from build123d import *

# Parameters (mm, degrees)
SKETCH_1_R          = 10.5
EXTRUDE_1_DEPTH     = 2.5
SKETCH_2_R          = 4.5
EXTRUDE_2_DEPTH     = 3
SKETCH_3_R          = 3
CUT_EXTRUDE_1_DEPTH = 3.5
SKETCH_4_R          = 0.75
CUT_EXTRUDE_2_DEPTH = 4


with BuildPart() as part:
    # 草图1 → 凸台-拉伸1 (new body)
    with BuildSketch(Plane(origin=(0, 0, 0), x_dir=(1, 0, 0), z_dir=(0, 1, 0))):
        with Locations(Location((0, 0, 0), (0, 0, 270))):
            Circle(SKETCH_1_R)
    extrude(amount=EXTRUDE_1_DEPTH)

    # 草图2 → 凸台-拉伸2 (add)
    with BuildSketch(Plane(origin=(0, 2.5, 0), x_dir=(1, 0, 0), z_dir=(0, 1, 0))):
        with Locations(Location((0, 0, 0), (0, 0, 270))):
            Circle(SKETCH_2_R)
    extrude(amount=EXTRUDE_2_DEPTH)

    # 草图3 → 切除-拉伸1 (cut)
    with BuildSketch(Plane(origin=(0, 5.5, 0), x_dir=(1, 0, 0), z_dir=(0, 1, 0))):
        with Locations(Location((0, 0, 0), (0, 0, 270))):
            Circle(SKETCH_3_R)
    extrude(amount=-CUT_EXTRUDE_1_DEPTH, mode=Mode.SUBTRACT)

    # 草图4 → 切除-拉伸2 (cut)
    with BuildSketch(Plane.XZ):
        with Locations(Location((0, 8, 0), (0, 0, 270))):
            Circle(SKETCH_4_R)
        with Locations(Location((3.253893145, 7.308363661, 0), (0, 0, 270))):
            Circle(SKETCH_4_R)
        with Locations(Location((5.945158604, 5.353044851, 0), (0, 0, 270))):
            Circle(SKETCH_4_R)
        with Locations(Location((7.60845213, 2.472135955, 0), (0, 0, 270))):
            Circle(SKETCH_4_R)
        with Locations(Location((7.956175163, -0.836227706, 0), (0, 0, 270))):
            Circle(SKETCH_4_R)
        with Locations(Location((6.92820323, -4, 0), (0, 0, 270))):
            Circle(SKETCH_4_R)
        with Locations(Location((4.702282018, -6.472135955, 0), (0, 0, 270))):
            Circle(SKETCH_4_R)
        with Locations(Location((1.663293527, -7.825180806, 0), (0, 0, 270))):
            Circle(SKETCH_4_R)
        with Locations(Location((-1.663293527, -7.825180806, 0), (0, 0, 270))):
            Circle(SKETCH_4_R)
        with Locations(Location((-4.702282018, -6.472135955, 0), (0, 0, 270))):
            Circle(SKETCH_4_R)
        with Locations(Location((-6.92820323, -4, 0), (0, 0, 270))):
            Circle(SKETCH_4_R)
        with Locations(Location((-7.956175163, -0.836227706, 0), (0, 0, 270))):
            Circle(SKETCH_4_R)
        with Locations(Location((-7.60845213, 2.472135955, 0), (0, 0, 270))):
            Circle(SKETCH_4_R)
        with Locations(Location((-5.945158604, 5.353044851, 0), (0, 0, 270))):
            Circle(SKETCH_4_R)
        with Locations(Location((-3.253893145, 7.308363661, 0), (0, 0, 270))):
            Circle(SKETCH_4_R)
    extrude(amount=-CUT_EXTRUDE_2_DEPTH, mode=Mode.SUBTRACT)


solid = part.part
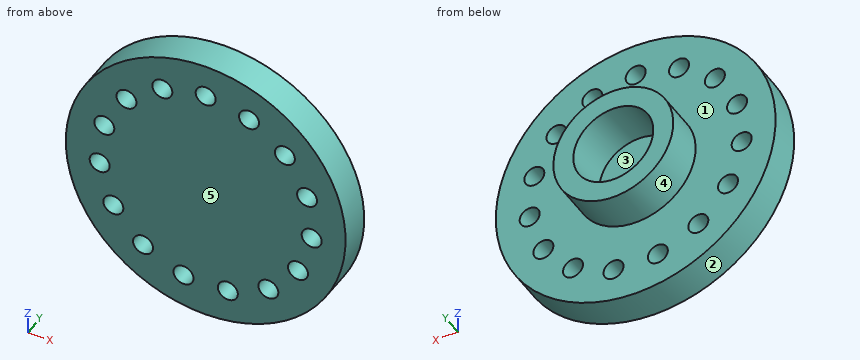
Can you work these out from the model? Positions are in its coordinate system, mm. Face numbers are marked on the shaded views. A direction names the side the tool comes from. Coordinates: 2 decimals unless noted, no trailing zeros. Write each loop counter-clockwise with the first axis right and the second up, starting at its lowest first coordinate (ties: lowest second). Pieces come first, ordered by that corner, then holes. Notation, with made-up numbers: (14.5, 15.5) -> (43.5, 15.5) arc R15 ccw to (43.5, 44.5) -> close; hole circle Ø4 at (-2, 74.25). An arc over 180 degrees is marked (long way). Write item = value, one per line.
(1) If I drill on probe 1 along Z at (x, y) = (-7, 0.3); probe 2 along X at (y, z) = (1.05, -3.5); probe 3 along Z at (x, y) = (5.5, 0.3), over which ranges is the centre line in solid material (lowest first)?
Verdict:
probe_1 = -7.83 to -4.75, -3.25 to 2.03, 2.91 to 7.83
probe_2 = -9.9 to -7.49, -6.37 to 6.37, 7.49 to 9.9
probe_3 = -8.94 to 4.75, 5.96 to 8.94
(2) On a 3-axis mill with a long thin cutter (end or side, diameter ignored), from which of +Z, -Z, +X, -X, +Y, -Y can I reach the whole of each face in a straight line? I mean the marked faces 4 and 5. Say none if no direction works.
Verdict:
face_4 = +Y
face_5 = +Z, -Z, +X, -X, -Y
(3) Thinking about a two-plate mould opening in Z: for the marked faces 1, 2 and 3, which applies, +Z half, -Z half, draft (parallel to the pull), parting line (faces both ways), or undercut?
Verdict:
face_1 = draft
face_2 = parting line
face_3 = undercut
(4) Imagine slicing it at D-D (z = 1). Please give me the cut outline in (x, y), and give its area (3 significant figures).
Verdict:
outline = (-10.45, 0) -> (10.45, 0) -> (10.45, 2.5) -> (4.39, 2.5) -> (4.39, 5.5) -> (2.83, 5.5) -> (2.83, 2) -> (-2.83, 2) -> (-2.83, 5.5) -> (-4.39, 5.5) -> (-4.39, 2.5) -> (-10.45, 2.5) -> close
area = 58.8 mm^2
(5) Imagine slicing it at C-C (y = 4.75). Please give me the cut outline in (x, z).
Verdict:
outline = circle Ø9 at (0, 0); hole circle Ø6 at (0, 0)
(6) Imagine slicing it at A-A (x = 0). Please give me the cut outline in (y, z).
Verdict:
outline = (0, -10.5) -> (2.5, -10.5) -> (2.5, -4.5) -> (5.5, -4.5) -> (5.5, -3) -> (2, -3) -> (2, 3) -> (5.5, 3) -> (5.5, 4.5) -> (2.5, 4.5) -> (2.5, 7.25) -> (0, 7.25) -> close; (0, 8.75) -> (2.5, 8.75) -> (2.5, 10.5) -> (0, 10.5) -> close
(7) Imagine slicing it at B-B (z = -4). Please give me the cut outline in (x, y).
Verdict:
outline = (-9.71, 0) -> (-7.68, 0) -> (-7.68, 2.5) -> (-9.71, 2.5) -> close; (-6.18, 0) -> (6.18, 0) -> (6.18, 2.5) -> (2.06, 2.5) -> (2.06, 5.5) -> (-2.06, 5.5) -> (-2.06, 2.5) -> (-6.18, 2.5) -> close; (7.68, 0) -> (9.71, 0) -> (9.71, 2.5) -> (7.68, 2.5) -> close
(8) For pin 1 (2 mm diameter, centred on y = 4.5, z = -4, fed in from -X); pin 2 (1.7 mm diameter, centred on x = -7.96, z = -0.84, fed in from +Y); pin 3 (2.5 mm diameter, centred on x = 1.66, z = -7.83, fed in from -Y); pin 4 (1.4 mm diameter, centred on x = -3.25, z = 7.31, fed in from -Y), each with a flat end and sliding along its axis, tell me the tip position at first contact or that it passes through.
Verdict:
pin_1 = -3.35
pin_2 = 2.5
pin_3 = 0
pin_4 = through
